```python
from build123d import *

# Parameters (mm, degrees)
F1_DEPTH = 1.2
F2_W     = 1.2
F2_H     = 40
F2_W_2   = 41.5
F2_H_2   = 1.2
F3_DEPTH = 10
F4_SIZE  = 0.4
F5_R     = 5
F6_DEPTH = 3
F7_SIZE  = 0.5


with BuildPart() as f1:
    # F0 (on Top) → F1 (new body)
    with BuildSketch(Plane.XY):
        with BuildLine():
            Line((44.5, 47.5), (3, 47.5))
            ThreePointArc((3, 47.5), (-0.181981, 46.181981), (-1.5, 43))
            Line((-1.5, 43), (-1.5, 3))
            ThreePointArc((-1.5, 3), (-0.181981, -0.181981), (3, -1.5))
            Line((3, -1.5), (44.5, -1.5))
            ThreePointArc((44.5, -1.5), (47.681981, -0.181981), (49, 3))
            Line((49, 3), (49, 43))
            ThreePointArc((49, 43), (47.681981, 46.181981), (44.5, 47.5))
        make_face()
        with BuildLine():
            Line((44.5, 0), (3, 0))
            ThreePointArc((3, 0), (0.87868, 0.87868), (0, 3))
            Line((0, 3), (0, 43))
            ThreePointArc((0, 43), (0.87868, 45.12132), (3, 46))
            Line((3, 46), (44.5, 46))
            ThreePointArc((44.5, 46), (46.62132, 45.12132), (47.5, 43))
            Line((47.5, 43), (47.5, 3))
            ThreePointArc((47.5, 3), (46.62132, 0.87868), (44.5, 0))
        make_face(mode=Mode.SUBTRACT)
        with BuildLine():
            ThreePointArc((0, 3), (0.87868, 0.87868), (3, 0))
            Line((3, 0), (44.5, 0))
            ThreePointArc((44.5, 0), (46.62132, 0.87868), (47.5, 3))
            Line((47.5, 3), (47.5, 43))
            ThreePointArc((47.5, 43), (46.62132, 45.12132), (44.5, 46))
            Line((44.5, 46), (3, 46))
            ThreePointArc((3, 46), (0.87868, 45.12132), (0, 43))
            Line((0, 43), (0, 3))
        make_face()
    extrude(amount=F1_DEPTH)

    # F2 (on face) → F3 (join)
    with BuildSketch(Plane.XY):
        with Locations((0.6, 23)):
            Rectangle(F2_W, F2_H)
        with Locations((46.9, 23)):
            Rectangle(F2_W, F2_H)
        with Locations((23.75, 0.6)):
            Rectangle(F2_W_2, F2_H_2)
        with Locations((23.75, 45.4)):
            Rectangle(F2_W_2, F2_H_2)
    extrude(amount=F3_DEPTH)

    # F4
    f4_edges = [f1.edges().sort_by_distance(p)[0] for p in [
        (47.5, 23, 10),
        (23.75, 46, 10),
        (0, 23, 10),
        (23.75, 0, 10),
    ]]
    chamfer(f4_edges, length=F4_SIZE)

    # F5
    f5_edges = [f1.edges().sort_by_distance(p)[0] for p in [
        (46.7, 43, 10),
        (44.5, 45.2, 10),
        (3, 45.2, 10),
        (0.8, 43, 10),
        (3, 0.8, 10),
        (0.8, 3, 10),
        (46.7, 3, 10),
        (44.5, 0.8, 10),
    ]]
    fillet(f5_edges, radius=F5_R)

    # F2 (on face) → F6 (join)
    with BuildSketch(Plane.XY):
        with BuildLine():
            Line((0, 43), (1.2, 43))
            ThreePointArc((1.2, 43), (1.727208, 44.272792), (3, 44.8))
            Line((3, 44.8), (3, 46))
            ThreePointArc((3, 46), (0.87868, 45.12132), (0, 43))
        make_face()
        with BuildLine():
            ThreePointArc((3, 1.2), (1.727208, 1.727208), (1.2, 3))
            Line((1.2, 3), (0, 3))
            ThreePointArc((0, 3), (0.87868, 0.87868), (3, 0))
            Line((3, 0), (3, 1.2))
        make_face()
        with BuildLine():
            ThreePointArc((46.3, 3), (45.772792, 1.727208), (44.5, 1.2))
            Line((44.5, 1.2), (44.5, 0))
            ThreePointArc((44.5, 0), (46.62132, 0.87868), (47.5, 3))
            Line((47.5, 3), (46.3, 3))
        make_face()
        with BuildLine():
            Line((44.5, 46), (44.5, 44.8))
            ThreePointArc((44.5, 44.8), (45.772792, 44.272792), (46.3, 43))
            Line((46.3, 43), (47.5, 43))
            ThreePointArc((47.5, 43), (46.62132, 45.12132), (44.5, 46))
        make_face()
    extrude(amount=F6_DEPTH)

    # F7
    f7_edges = [f1.edges().sort_by_distance(p)[0] for p in [
        (49, 23, 0),
        (47.681981, 46.181981, 0),
        (23.75, 47.5, 0),
        (-0.181981, 46.181981, 0),
        (-1.5, 23, 0),
        (-0.181981, -0.181981, 0),
        (23.75, -1.5, 0),
        (47.681981, -0.181981, 0),
    ]]
    chamfer(f7_edges, length=F7_SIZE)


solid = f1.part
```
Source: CAD feature listing. Evaluate the final solid. Frame: model axes, mm. A direction names the side the tool comes from. Coordinates: 2 decimals unless noted, no trailing zeros. Loops run counter-clockwise (first coordinate to the right, second up) from the corner with the lowest first, then second, coordinate; pieces in that order, holes last. Notation, with made-up numbers: M -39,0.25 L -27,0.25 A30 ccw -27,37.25 Z; hole C -10.75,53.25 d8. An arc over 180 degrees is marked long. Use a Markdown table: item, result. Add a question column.
Q1. Draft query along X for faces 6 (the cylindrical face through (1.713, 44.259, 2.087)), 7 (the flat face through (47, 3, 4)), 8 (the conical face through (47.397, 0.039, 0.142)). Return one class per face: pulls with the +X half, pulls with the -X half, needs draft (parallel to the pull), parting line crosses it, or undercut.
Q2. Material intervals for L1, parallel to X at y = 22, z = 2.25; L2, parallel to Y at x = 42, z = 5.5; L3, parallel to Z at x = 3, y = 37.5, sorted ascending.
Q3. First-contact query: pin 1 (1.3 mm diameter, centred on x = 0.5, z = 4.5, fed in from +Y); pin 2 (5 mm diameter, centred on y = 22.5, z = 4, fed in from -X); pin 3 (2.5 mm diameter, centred on x = 46, y = 45, fed in from +Z). Flat tips, straight axial feed; report the tip coordinate or a pass-through.
Q4. Section query A-A, the plane z = 9. Return loops of the section in (x, y), and give its area (3 significant figures).
Q5. Section query B-B, the plane x = 18.5. Return loops of the section in (y, z).
Q6. Section query D-D, the plane z = 5.75. Return loops of the section in (x, y), and give its area (3 significant figures).
Q7. Access query for faces 1 (the cylindrical face through (0.86, 0.9, 2.09)), 2 (the cylindrical face through (45.787, 1.741, 2.087)), 3 (the flat face through (23, 0, 5)), 4 (the flat face through (3, 45, 4)), 5 (the cylindrical face through (46.6, 0.86, 2.09)). Directions: +Z, -Z, +X, -X, +Y, -Y. A direction counts if a zero-diameter tool reaches every point of the face in a straight line with its end or side. Return the directions, or none.
Q8. Section query C-C, the plane y = 25. Return loops of the section in (x, z), and give its area (3 significant figures).
Result:
| question | item | result |
|---|---|---|
| 1 | face 6 | undercut |
| 1 | face 7 | needs draft |
| 1 | face 8 | pulls with the +X half |
| 2 | L1 | x = 0 to 1.2, 46.3 to 47.5 |
| 2 | L2 | y = 0 to 1.2, 44.8 to 46 |
| 2 | L3 | z = 0 to 1.2 |
| 3 | pin 1 | stops at y = 43 |
| 3 | pin 2 | stops at x = 0 |
| 3 | pin 3 | stops at z = 3 |
| 4 | outline | M 0,5 L 1.2,5 L 1.2,41 L 0,41 Z; M 5,0 L 42.5,0 L 42.5,1.2 L 5,1.2 Z; M 5,44.8 L 42.5,44.8 L 42.5,46 L 5,46 Z; M 46.3,5 L 47.5,5 L 47.5,41 L 46.3,41 Z |
| 4 | area | 176 mm2 |
| 5 | outline | M -1.5,0.5 L -1,0 L 47,0 L 47.5,0.5 L 47.5,1.2 L 46,1.2 L 46,9.6 L 45.6,10 L 44.8,10 L 44.8,1.2 L 1.2,1.2 L 1.2,10 L 0.4,10 L 0,9.6 L 0,1.2 L -1.5,1.2 Z |
| 6 | outline | M 0,3.06 L 1.2,3.06 L 1.2,42.94 L 0,42.94 Z; M 3.06,0 L 44.44,0 L 44.44,1.2 L 3.06,1.2 Z; M 3.06,44.8 L 44.44,44.8 L 44.44,46 L 3.06,46 Z; M 46.3,3.06 L 47.5,3.06 L 47.5,42.94 L 46.3,42.94 Z |
| 6 | area | 195 mm2 |
| 7 | face 1 | +Z, -X, -Y |
| 7 | face 2 | +Z |
| 7 | face 3 | +Z, +X, -X, -Y |
| 7 | face 4 | +Z, -X, +Y, -Y |
| 7 | face 5 | +Z, +X, -Y |
| 8 | outline | M -1.5,0.5 L -1,0 L 48.5,0 L 49,0.5 L 49,1.2 L 47.5,1.2 L 47.5,9.6 L 47.1,10 L 46.3,10 L 46.3,1.2 L 1.2,1.2 L 1.2,10 L 0.4,10 L 0,9.6 L 0,1.2 L -1.5,1.2 Z |
| 8 | area | 81.3 mm2 |
